```python
from build123d import *

# Parameters (mm, degrees)
EXTRUSION1_DEPTH = 15
ESQUISSE3_R      = 1.5
EXTRUSION2_DEPTH = 40
ESQUISSE5_R      = 1.5
ESQUISSE5_W      = 7
ESQUISSE5_H      = 4
EXTRUSION3_DEPTH = 40


with BuildPart() as part:
    # Esquisse1 → Extrusion1 (new body)
    with BuildSketch(Plane(origin=(0, 0, 0), x_dir=(1, 0, 0), z_dir=(0, 1, 0))):
        Polygon((5.12562835, -15.59067149), (-14.87437165, -15.59067149), (-14.87437165, 4.40932851), (-13.37437165, 4.40932851), (-13.37437165, -14.09067149), (5.12562835, -14.09067149), align=None)
    extrude(amount=EXTRUSION1_DEPTH)

    # Esquisse3 → Extrusion2 (cut)
    with BuildSketch(Plane(origin=(0, 0, 14.09067149), x_dir=(-1, 0, 0), z_dir=(0, 0, -1))):
        with Locations((2.87437165, 5)):
            Circle(ESQUISSE3_R)
        with Locations((9.87437165, 5)):
            Circle(ESQUISSE3_R)
    extrude(amount=-EXTRUSION2_DEPTH, mode=Mode.SUBTRACT)

    # Esquisse5 → Extrusion3 (cut)
    with BuildSketch(Plane(origin=(-13.37437165, 0, 0), x_dir=(0, 0, -1), z_dir=(1, 0, 0))):
        with Locations((-6.59067149, 4)):
            Circle(ESQUISSE5_R)
        with Locations((-6.59067149, 11)):
            Circle(ESQUISSE5_R)
        with Locations((1.90932851, 7.5)):
            Rectangle(ESQUISSE5_W, ESQUISSE5_H)
    extrude(amount=-EXTRUSION3_DEPTH, mode=Mode.SUBTRACT)


solid = part.part
```
CAD build for the part. Positions are in the model's coordinates, mm. A direction names the side the tool comes from. Coordinates: 2 decimals unless noted, no trailing zeros. Write each loop counter-clockwise with the first axis right and the second up, starting at its lowest first coordinate (ties: lowest second). Pieces come first, ordered by that corner, then holes. Notation, with made-up numbers: (-34, 28.5) -> (5, 28.5) arc R17 ccw to (5, 38.5) -> close; hole circle Ø2 at (73.25, 18). An arc over 180 degrees is marked (long way). Return JSON: item names as keys, results as strings. Group by question number.
Q1. Drill centre lines: line 1 (Y direction, x = -13.5, z = 7.5); line 2 (Z direction, x = -5.75, y = 14.5); line 3 (X direction, y = 13.75, z = 12.75). Where is each one in solid material? Low to high.
Q2. Flat gauge pins, fed straight in: pin 1 (6 mm diameter, centred on x = -9, z = -0.5, fed in from +Y); pin 2 (5 mm diameter, centred on y = 5.5, z = -1, fed in from +X); pin 3 (4.5 mm diameter, centred on x = -3, y = 7, fed in from -Z); pin 4 (0.8 mm diameter, centred on x = -14, y = 8, fed in from -Z). Where does each tip first touch, or does it go through?
Q3. Cut at A-A, the plane y = 11. Give the cut face in (x, z).
Q4. Cut at B-B, the plane z = 0. Give the cut face in (x, y), then the cut area to 3 significant figures.
Q5. Cut at D-D, the plane y = 8.25. Give the cut face in (x, z), then the cut area to 4 significant figures.
Q6. Pull direction X, two halves, no side cores. Call faces 4 (the face through (-14, 7, 1.591)), 5 (the face through (-11.26, 4.43, 14.83)), 6 (the face through (-4.305, 5.451, 14.83)), 7 (the face through (5.126, 7, 15)): released by +X, released by -X, zero draft, split by the parting line, or undercut.
Q7. Which spindle directions (+Z, -Z, +X, -X, +Y, -Y) get a long thin tool onto all of the face, cutting with end or side? Do faces 1 (the face through (-14, 5.5, -1)), 2 (the face through (-4, 7, 14.091)), 3 (the face through (-14, 12, -4.409)). Say none if no direction does.
Q8. Cut at C-C, the plane x = -3.5. Give the cut face in (y, z).
Returned:
{
 "1": {"line 1": "y = 0 to 2.81, 5.19 to 9.81, 12.19 to 15", "line 2": "z = 14.09 to 15.59", "line 3": "x = -14.87 to -13.37"},
 "2": {"pin 1": "passes through", "pin 2": "stops at x = -13.37", "pin 3": "stops at z = 14.09", "pin 4": "stops at z = 1.59"},
 "3": {"outline": "(-14.87, -4.41) -> (-13.37, -4.41) -> (-13.37, 5.09) -> (-14.87, 5.09) -> close; (-14.87, 8.09) -> (-13.37, 8.09) -> (-13.37, 14.09) -> (5.13, 14.09) -> (5.13, 15.59) -> (-14.87, 15.59) -> close"},
 "4": {"outline": "(-14.87, 0) -> (-13.37, 0) -> (-13.37, 5.5) -> (-14.87, 5.5) -> close; (-14.87, 9.5) -> (-13.37, 9.5) -> (-13.37, 15) -> (-14.87, 15) -> close", "area": "16.5 mm2"},
 "5": {"outline": "(-14.87, 1.59) -> (-13.37, 1.59) -> (-13.37, 14.09) -> (5.13, 14.09) -> (5.13, 15.59) -> (-14.87, 15.59) -> close", "area": "48.75 mm2"},
 "6": {"face 4": "zero draft", "face 5": "undercut", "face 6": "undercut", "face 7": "released by +X"},
 "7": {"face 1": "-Z, +X, -X", "face 2": "-Z, +X, +Y, -Y", "face 3": "-Z, +X, -X, +Y, -Y"},
 "8": {"outline": "(0, 14.09) -> (3.64, 14.09) -> (3.64, 15.59) -> (0, 15.59) -> close; (6.36, 14.09) -> (15, 14.09) -> (15, 15.59) -> (6.36, 15.59) -> close"}
}
